Design review of the part built by this model. Coordinates are the model's own, in mm. Face numbers are marked on the shaded views. A direction names the side the tool comes from. Give positions to 0.01 mm unless a question says otherwise; leave off trailing zeros. Loops run counter-clockwise (first coordinate to the right, second up) from the corner with the lowest first, then second, coordinate; pieces in that order, holes last. Notation, with made-up numbers: M 86.5,89 L 139.5,89 A5 ccw 139.5,93 Z; hole C 40,79.25 d10. An arc over 180 degrees is marked long. Answer as CSV lines item,"result".
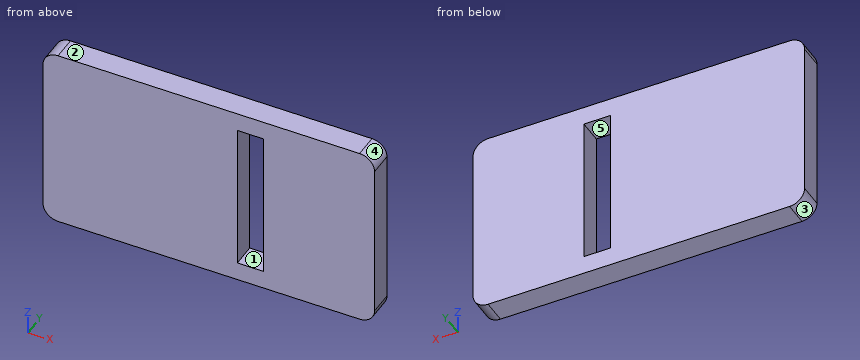
```python
from build123d import *

# Parameters (mm, degrees)
SKETCH1_W           = 88.18
SKETCH1_H           = 50
SKETCH1_W_2         = 7
SKETCH1_H_2         = 40
BOSS_EXTRUDE1_DEPTH = 6.35
FILLET1_R           = 4


with BuildPart() as part:
    # Sketch1 → Boss-Extrude1 (new body)
    with BuildSketch(Plane(origin=(0, 0, 0), x_dir=(1, 0, 0), z_dir=(0, 1, 0))):
        Rectangle(SKETCH1_W, SKETCH1_H)
        with Locations((11.09, 0)):
            Rectangle(SKETCH1_W_2, SKETCH1_H_2, mode=Mode.SUBTRACT)
    extrude(amount=BOSS_EXTRUDE1_DEPTH)

    # Fillet1
    fillet1_edges = [part.edges().sort_by_distance(p)[0] for p in [
        (44.09, 3.175, 25),
        (-44.09, 3.175, 25),
        (-44.09, 3.175, -25),
        (44.09, 3.175, -25),
    ]]
    fillet(fillet1_edges, radius=FILLET1_R)


solid = part.part
```
1. The part is to be moulded in two halves that separate along X. For the marked faces 3, 4 and 5, say which applies: pulls with the +X half, pulls with the -X half, needs draft (parallel to the pull), parting line crosses it, or undercut.
Answer block:
face 3,"pulls with the -X half"
face 4,"pulls with the +X half"
face 5,"undercut"
2. We need section A-A, the plane x = 8.5. Write out the cut boundary in (y, z).
Answer block:
outline,"M 0,-25 L 6.35,-25 L 6.35,-20 L 0,-20 Z; M 0,20 L 6.35,20 L 6.35,25 L 0,25 Z"
3. For the marked faces 1 and 2, list the 3-axis set-ups (+Z, -Z, +X, -X, +Y, -Y) from which the entire face can be reached by the end or side of a thin tool; tool diameter is ignored.
Answer block:
face 1,"+Y, -Y"
face 2,"+Z, +X, -X, +Y, -Y"
4. For P1, Ø4, axis at x = 12.5, z = 17.5, coming from the +Y side, flat-tipped, find the tip position at first contact; note if it passes through.
Answer block:
P1,"through"
5. To check wall thickness, follow L1, parallel to X at y = 3.75, z = 3.5; L2, parallel to Z at x = 8.5, y = 5.5; L3, parallel to X at y = 4, z = 22. State the ranges of each line that lie inside material, in increasing order. Write a range as [from, to].
Answer block:
L1,"[-44.09, 7.59], [14.59, 44.09]"
L2,"[-25, -20], [20, 25]"
L3,"[-43.96, 43.96]"
6. We need section B-B, the plane z = -14.5. Write out the cut boundary in (x, y), plus the area to 3 significant figures.
Answer block:
outline,"M -44.09,0 L 7.59,0 L 7.59,6.35 L -44.09,6.35 Z; M 14.59,0 L 44.09,0 L 44.09,6.35 L 14.59,6.35 Z"
area,"515 mm²"
7. We need section C-C, the plane y = 2.5. Write out the cut boundary in (x, z), plus the area to 3 significant figures.
Answer block:
outline,"M -44.09,-21 A4 ccw -40.09,-25 L 40.09,-25 A4 ccw 44.09,-21 L 44.09,21 A4 ccw 40.09,25 L -40.09,25 A4 ccw -44.09,21 Z; hole M 7.59,-20 L 14.59,-20 L 14.59,20 L 7.59,20 Z"
area,"4,120 mm²"
